Input: part model. Units: mm. Frame: model coordinates. Coordinates: 2 decimals unless noted, no trailing zeros. Write each loop counter-clockwise with the first axis right and the second up, starting at its lowest first coordinate (ties: lowest second). Pieces come first, ordered by that corner, then holes. Notation, with made-up numbers: (28.5, 52) - (63.5, 52) arc R31 cw to (63.5, 80) - close; hole circle Ø10 at (-30.75, 37.25). An arc over 180 degrees is marked (long way). Use CSV: the item, a comma, the result in double quotes.
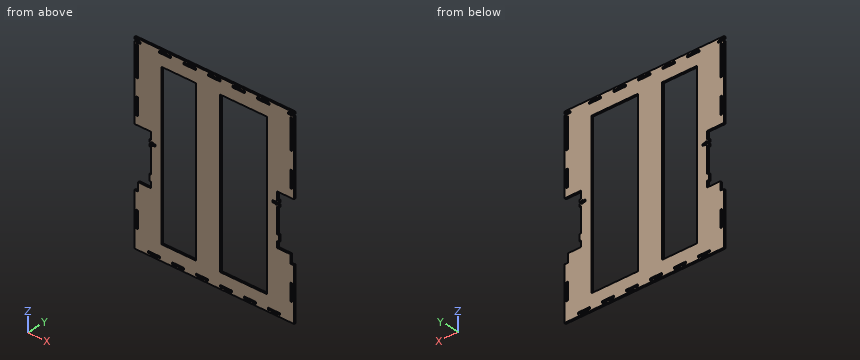
```python
from build123d import *

# Parameters (mm, degrees)
SKETCH1_W           = 3
SKETCH1_H           = 49.4545
SKETCH1_W_2         = 20.4615
SKETCH1_H_2         = 3
SKETCH1_H_3         = 27.7273
SKETCH1_W_3         = 20
SKETCH1_W_4         = 176
SKETCH1_H_4         = 261
BOSS_EXTRUDE1_DEPTH = 3
SKETCH2_W           = 10.5
SKETCH2_H           = 3.2
SKETCH2_W_2         = 2.5
SKETCH2_H_2         = 5.2
CUT_EXTRUDE1_DEPTH  = 10
SKETCH4_W           = 40
SKETCH4_H           = 261
BOSS_EXTRUDE2_DEPTH = 3


with BuildPart() as part:
    # Sketch1 → Boss-Extrude1 (new body)
    with BuildSketch(Plane(origin=(0, 0, 0), x_dir=(1, 0, 0), z_dir=(0, 1, 0))):
        Polygon((-133, -152.5), (-133, -155.5), (133, -155.5), (133, -152.5), (123, -152.5), (123, -149.5), (133, -149.5), (133, -27.7273), (105, -27.7273), (105, -15.2273), (108, -15.2273), (108, -5.2273), (105, -5.2273), (105, 35.4545), (108, 35.4545), (108, 45.4545), (105, 45.4545), (105, 55.4545), (127, 55.4545), (127, 69.3181), (133, 69.3181), (133, 155.5), (-133, 155.5), (-133, 69.3181), (-127, 69.3181), (-127, 55.4545), (-105, 55.4545), (-105, 45.4545), (-108, 45.4545), (-108, 35.4545), (-105, 35.4545), (-105, -5.2273), (-108, -5.2273), (-108, -15.2273), (-105, -15.2273), (-105, -27.7273), (-133, -27.7273), (-133, -149.5), (-123, -149.5), (-123, -152.5), align=None)
        with Locations((-128.5, -121.77275)):
            Rectangle(SKETCH1_W, SKETCH1_H, mode=Mode.SUBTRACT)
        with Locations((-81.846, -151)):
            Rectangle(SKETCH1_W_2, SKETCH1_H_2, mode=Mode.SUBTRACT)
        with Locations((-40.923, -151)):
            Rectangle(SKETCH1_W_2, SKETCH1_H_2, mode=Mode.SUBTRACT)
        with Locations((0, -151)):
            Rectangle(SKETCH1_W_2, SKETCH1_H_2, mode=Mode.SUBTRACT)
        with Locations((-128.5, -55.45455)):
            Rectangle(SKETCH1_W, SKETCH1_H_3, mode=Mode.SUBTRACT)
        with Locations((40.923, -151)):
            Rectangle(SKETCH1_W_2, SKETCH1_H_2, mode=Mode.SUBTRACT)
        with Locations((81.846, -151)):
            Rectangle(SKETCH1_W_2, SKETCH1_H_2, mode=Mode.SUBTRACT)
        with Locations((128.5, -121.77275)):
            Rectangle(SKETCH1_W, SKETCH1_H, mode=Mode.SUBTRACT)
        with Locations((128.5, -55.45455)):
            Rectangle(SKETCH1_W, SKETCH1_H_3, mode=Mode.SUBTRACT)
        with Locations((-128.5, 110.90905)):
            Rectangle(SKETCH1_W, SKETCH1_H_3, mode=Mode.SUBTRACT)
        with Locations((-100, 151)):
            Rectangle(SKETCH1_W_3, SKETCH1_H_2, mode=Mode.SUBTRACT)
        with Locations((-60, 151)):
            Rectangle(SKETCH1_W_3, SKETCH1_H_2, mode=Mode.SUBTRACT)
        with Locations((-20, 151)):
            Rectangle(SKETCH1_W_3, SKETCH1_H_2, mode=Mode.SUBTRACT)
        Rectangle(SKETCH1_W_4, SKETCH1_H_4, mode=Mode.SUBTRACT)
        with Locations((20, 151)):
            Rectangle(SKETCH1_W_3, SKETCH1_H_2, mode=Mode.SUBTRACT)
        with Locations((60, 151)):
            Rectangle(SKETCH1_W_3, SKETCH1_H_2, mode=Mode.SUBTRACT)
        with Locations((128.5, 110.90905)):
            Rectangle(SKETCH1_W, SKETCH1_H_3, mode=Mode.SUBTRACT)
        with Locations((100, 151)):
            Rectangle(SKETCH1_W_3, SKETCH1_H_2, mode=Mode.SUBTRACT)
    extrude(amount=BOSS_EXTRUDE1_DEPTH)

    # Sketch2 → Cut-Extrude1 (cut)
    with BuildSketch(Plane(origin=(0, 3, 0), x_dir=(1, 0, 0), z_dir=(0, 1, 0))):
        with Locations((-102.75, -10.2273)):
            Rectangle(SKETCH2_W, SKETCH2_H)
        with Locations((102.75, -10.2273)):
            Rectangle(SKETCH2_W, SKETCH2_H)
        with Locations((103.575, -10.2273)):
            Rectangle(SKETCH2_W_2, SKETCH2_H_2)
        with Locations((-103.575, -10.2273)):
            Rectangle(SKETCH2_W_2, SKETCH2_H_2)
    extrude(amount=-CUT_EXTRUDE1_DEPTH, mode=Mode.SUBTRACT)

    # Sketch4 → Boss-Extrude2 (add)
    with BuildSketch(Plane(origin=(0, 0, 0), x_dir=(1, 0, 0), z_dir=(0, 1, 0))):
        with Locations((-10, 0)):
            Rectangle(SKETCH4_W, SKETCH4_H)
    extrude(amount=BOSS_EXTRUDE2_DEPTH)


solid = part.part
```
(1) Cut plane A-A on z = 50. Return loops of the section in (x, y).
Check values:
outline,"(-133, 0) - (-130, 0) - (-130, 3) - (-133, 3) - close; (-127, 0) - (-88, 0) - (-88, 3) - (-127, 3) - close; (-30, 0) - (10, 0) - (10, 3) - (-30, 3) - close; (88, 0) - (127, 0) - (127, 3) - (88, 3) - close; (130, 0) - (133, 0) - (133, 3) - (130, 3) - close"
(2) Cut plane B-B on x = 59.5. Return loops of the section in (y, z).
Check values:
outline,"(0, -155.5) - (3, -155.5) - (3, -152.5) - (0, -152.5) - close; (0, -149.5) - (3, -149.5) - (3, -130.5) - (0, -130.5) - close; (0, 130.5) - (3, 130.5) - (3, 155.5) - (0, 155.5) - close"
(3) Cut plane C-C on z = -18. Return loops of the section in (x, y).
Check values:
outline,"(-105, 0) - (-88, 0) - (-88, 3) - (-105, 3) - close; (-30, 0) - (10, 0) - (10, 3) - (-30, 3) - close; (88, 0) - (105, 0) - (105, 3) - (88, 3) - close"
(4) Pin query (flat end, axial travel): pin 1 Ø1.5 at (y, z) = (1, 150.5) entering from +X; pin 2 Ø1.5 at (y, z) = (0.5, -54.5) entering from -X. Return the tip coordinate at first contact, or that it passes through.
Check values:
pin 1,"x = 123"
pin 2,"x = -105"
(5) Cut plane D-D on y = 1.6. State how many separate pieces and enclosed holes the cut face has, and give its area (3 significant figures).
Check values:
separate pieces,"1"
enclosed holes,"19"
area,"41,100 mm^2"
(6) Ray query, probe 1 along X at (y, z) = (1, -56.5); probe 2 along X at (y, z) = (0.4, -95.5); probe 3 along Z at (x, y) = (-55.5, 2.75). Return the intervals inside material, ascending. Write a range as from..to.
Check values:
probe 1,"-127..-88, -30..10, 88..127"
probe 2,"-133..-88, -30..10, 88..133"
probe 3,"-155.5..-152.5, -149.5..-130.5, 130.5..155.5"
